Read the model definition and answer for the solid it produces. Units are mm, in the model's axes. Face numbers are marked on the shaded views. A direction names the side the tool comes from. Give positions to 0.01 mm unless a question says otherwise; leave off trailing zeros. Write each loop counter-clockwise with the first axis right and the second up, starting at its lowest first coordinate (ties: lowest second). Pieces come first, ordered by that corner, then holes. Notation, with made-up numbers: M -7.5,19 L 22.5,19 A31 ccw 22.5,43 Z; hole C -24.75,-7.5 d10. An arc over 180 degrees is marked long. Use a Markdown table: item, result. Add a question column.
Item 1: Consider probe 1 along Y at (x, z) = (0, 6) (3 decimals); probe 2 along Z at (x, y) = (0, -11.7) (3 decimals); probe 3 along Y at (x, z) = (-11.5, 8). Determine where each line is inside the solid, lowest interval first. Write a range as [from, to].
Item 2: Given P1, Ø2.5, axis at x = 0, z = 7.125, coming from the +Y side; P2, Ø3, axis at y = -7.5, z = 5.5, coming from the +X side; P3, Ø2.5, axis at x = -4.5, z = 6, coming from the -Y side; P4, Ø3, axis at x = -3.5, y = -8.5, coming from the -Z side, each flat-ended and moving along its own axis, determine where each tip first touches the part or whether it passes through.
Item 3: For the marked faces 4 and 5, determine the directions among +Z, -Z, +X, -X, +Y, -Y from which every point of the face is accessible in a straight line to the end or side of a thin tool.
Item 4: The mould has two halves that part along Z. Classify the marked faces 1, 2 and 3: pulls with the +Z half, pulls with the -Z half, needs draft (parallel to the pull), parting line crosses it, or undercut.
Item 5: A cutting plane is placed at A-A on x = 0. Determine the outline of the cut face in (y, z) (3 decimals).
Item 6: A cutting plane is placed at B-B on z = 5.5. Determine the outline of the cut face in (x, y) (3 decimals).
Item 7: A cutting plane is placed at D-D on y = -4. Determine the outline of the cut face in (x, z).
Item 8: A cutting plane is placed at C-C on y = -11.75. Determine the outline of the cut face in (x, z) (3 decimals).
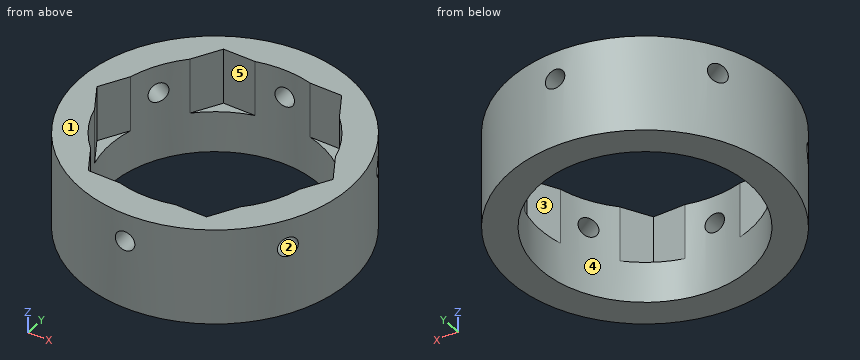
from build123d import *

# Parameters (mm, degrees)
SKETCH1_R               = 14
BOSS_EXTRUDE1_DEPTH     = 10
CUT_EXTRUDE1_REACH      = 24.181
SKETCH2_R               = 10.875
CUT_EXTRUDE2_DEPTH      = 5.75
CUT_EXTRUDE3_REACH      = 31.937
CUT_EXTRUDE3_END_RADIUS = 14
SKETCH4_R               = 1
CUT_EXTRUDE4_REACH      = 33.684
CUT_EXTRUDE4_END_RADIUS = 14
SKETCH5_R               = 1
CUT_EXTRUDE5_REACH      = 33.684
CUT_EXTRUDE5_END_RADIUS = 14
SKETCH6_R               = 1
CUT_EXTRUDE6_REACH      = 31.937
CUT_EXTRUDE6_END_RADIUS = 14
SKETCH7_R               = 1
CUT_EXTRUDE7_REACH      = 33.684
CUT_EXTRUDE7_END_RADIUS = 14
SKETCH8_R               = 1
CUT_EXTRUDE8_REACH      = 33.684
CUT_EXTRUDE8_END_RADIUS = 14
SKETCH9_R               = 1


with BuildPart() as part:
    # Sketch1 → Boss-Extrude1 (new body)
    with BuildSketch(Plane.XY):
        Circle(SKETCH1_R)
    extrude(amount=BOSS_EXTRUDE1_DEPTH)

    # Sketch2 → Cut-Extrude1 (cut, up to next)
    with BuildSketch(Plane.XY.offset(10), mode=Mode.PRIVATE) as cut_extrude1_sk1:
        Circle(SKETCH2_R)
    cut_extrude1_tool1 = extrude(cut_extrude1_sk1.sketch, amount=-CUT_EXTRUDE1_REACH, mode=Mode.PRIVATE) & part.part
    add(cut_extrude1_tool1.solids().sort_by_distance((0, 0, 10))[0], mode=Mode.SUBTRACT)

    # Sketch3 → Cut-Extrude2 (cut)
    with BuildSketch(Plane.XY.offset(10)):
        Polygon((12.124355653, 0), (6.062177826, 10.5), (-6.062177826, 10.5), (-12.124355653, 0), (-6.062177826, -10.5), (6.062177826, -10.5), align=None)
    extrude(amount=-CUT_EXTRUDE2_DEPTH, mode=Mode.SUBTRACT)

    # Cut-Extrude3: up to this cylinder (the profile starts inside it)
    cut_extrude3_end = Plane(origin=(0, 0, 7.125), z_dir=(0, 0, -1)) * Cylinder(CUT_EXTRUDE3_END_RADIUS, 92.874, mode=Mode.PRIVATE)
    # Sketch4 → Cut-Extrude3 (cut, up to the surface)
    with BuildSketch(Plane(origin=(0, 10.5, 0), x_dir=(-1, 0, 0), z_dir=(0, -1, 0)), mode=Mode.PRIVATE) as cut_extrude3_sk1:
        with Locations(Location((0, -7.125, 0), (0, 0, 180))):
            Circle(SKETCH4_R)
    cut_extrude3_tool1 = extrude(cut_extrude3_sk1.sketch, amount=-CUT_EXTRUDE3_REACH, mode=Mode.PRIVATE) & cut_extrude3_end
    add(cut_extrude3_tool1.solids().sort_by_distance((0, 10.5, 7.125))[0], mode=Mode.SUBTRACT)

    # Cut-Extrude4: up to this cylinder (the profile starts inside it)
    cut_extrude4_end = Plane(origin=(0, 0, 7.125), z_dir=(0, 0, -1)) * Cylinder(CUT_EXTRUDE4_END_RADIUS, 96.368, mode=Mode.PRIVATE)
    # Sketch5 → Cut-Extrude4 (cut, up to the surface)
    with BuildSketch(Plane(origin=(9.09326674, 5.25, 0), x_dir=(0, 0, 1), z_dir=(-0.8660254037844386, -0.4999999999999999, 0)), mode=Mode.PRIVATE) as cut_extrude4_sk1:
        with Locations(Location((7.125, 0, 0), (0, 0, 270))):
            Circle(SKETCH5_R)
    cut_extrude4_tool1 = extrude(cut_extrude4_sk1.sketch, amount=-CUT_EXTRUDE4_REACH, mode=Mode.PRIVATE) & cut_extrude4_end
    add(cut_extrude4_tool1.solids().sort_by_distance((9.093267, 5.25, 7.125))[0], mode=Mode.SUBTRACT)

    # Cut-Extrude5: up to this cylinder (the profile starts inside it)
    cut_extrude5_end = Plane(origin=(0, 0, 7.125), z_dir=(0, 0, -1)) * Cylinder(CUT_EXTRUDE5_END_RADIUS, 96.368, mode=Mode.PRIVATE)
    # Sketch6 → Cut-Extrude5 (cut, up to the surface)
    with BuildSketch(Plane(origin=(9.09326674, -5.25, 0), x_dir=(0, 0, 1), z_dir=(-0.8660254037844386, 0.5, 0)), mode=Mode.PRIVATE) as cut_extrude5_sk1:
        with Locations(Location((7.125, 0, 0), (0, 0, 270))):
            Circle(SKETCH6_R)
    cut_extrude5_tool1 = extrude(cut_extrude5_sk1.sketch, amount=-CUT_EXTRUDE5_REACH, mode=Mode.PRIVATE) & cut_extrude5_end
    add(cut_extrude5_tool1.solids().sort_by_distance((9.093267, -5.25, 7.125))[0], mode=Mode.SUBTRACT)

    # Cut-Extrude6: up to this cylinder (the profile starts inside it)
    cut_extrude6_end = Plane(origin=(0, 0, 7.125), z_dir=(0, 0, -1)) * Cylinder(CUT_EXTRUDE6_END_RADIUS, 92.874, mode=Mode.PRIVATE)
    # Sketch7 → Cut-Extrude6 (cut, up to the surface)
    with BuildSketch(Plane(origin=(0, -10.5, 0), x_dir=(1, 0, 0), z_dir=(0, 1, 0)), mode=Mode.PRIVATE) as cut_extrude6_sk1:
        with Locations((0, -7.125)):
            Circle(SKETCH7_R)
    cut_extrude6_tool1 = extrude(cut_extrude6_sk1.sketch, amount=-CUT_EXTRUDE6_REACH, mode=Mode.PRIVATE) & cut_extrude6_end
    add(cut_extrude6_tool1.solids().sort_by_distance((0, -10.5, 7.125))[0], mode=Mode.SUBTRACT)

    # Cut-Extrude7: up to this cylinder (the profile starts inside it)
    cut_extrude7_end = Plane(origin=(0, 0, 7.125), z_dir=(0, 0, -1)) * Cylinder(CUT_EXTRUDE7_END_RADIUS, 96.368, mode=Mode.PRIVATE)
    # Sketch8 → Cut-Extrude7 (cut, up to the surface)
    with BuildSketch(Plane(origin=(-9.09326674, -5.25, 0), x_dir=(0, 0, -1), z_dir=(0.8660254037844385, 0.5000000000000003, 0)), mode=Mode.PRIVATE) as cut_extrude7_sk1:
        with Locations(Location((-7.125, 0, 0), (0, 0, 270))):
            Circle(SKETCH8_R)
    cut_extrude7_tool1 = extrude(cut_extrude7_sk1.sketch, amount=-CUT_EXTRUDE7_REACH, mode=Mode.PRIVATE) & cut_extrude7_end
    add(cut_extrude7_tool1.solids().sort_by_distance((-9.093267, -5.25, 7.125))[0], mode=Mode.SUBTRACT)

    # Cut-Extrude8: up to this cylinder (the profile starts inside it)
    cut_extrude8_end = Plane(origin=(0, 0, 7.125), z_dir=(0, 0, -1)) * Cylinder(CUT_EXTRUDE8_END_RADIUS, 96.368, mode=Mode.PRIVATE)
    # Sketch9 → Cut-Extrude8 (cut, up to the surface)
    with BuildSketch(Plane(origin=(-9.09326674, 5.25, 0), x_dir=(0, 0, -1), z_dir=(0.8660254037844388, -0.49999999999999983, 0)), mode=Mode.PRIVATE) as cut_extrude8_sk1:
        with Locations(Location((-7.125, 0, 0), (0, 0, 270))):
            Circle(SKETCH9_R)
    cut_extrude8_tool1 = extrude(cut_extrude8_sk1.sketch, amount=-CUT_EXTRUDE8_REACH, mode=Mode.PRIVATE) & cut_extrude8_end
    add(cut_extrude8_tool1.solids().sort_by_distance((-9.093267, 5.25, 7.125))[0], mode=Mode.SUBTRACT)


solid = part.part
Filled in:
| question | item | result |
|---|---|---|
| 1 | probe 1 | [-14, -10.875], [10.875, 14] |
| 1 | probe 2 | [0, 6.125], [8.125, 10] |
| 1 | probe 3 | [-7.98, -7.2], [-6.08, -1.08], [1.08, 6.08], [7.2, 7.98] |
| 2 | P1 | y = 14 |
| 2 | P2 | x = 12.65 |
| 2 | P3 | y = -13.62 |
| 2 | P4 | through |
| 3 | face 4 | +Z, -Z |
| 3 | face 5 | +Z |
| 4 | face 1 | pulls with the +Z half |
| 4 | face 2 | undercut |
| 4 | face 3 | needs draft |
| 5 | outline | M -14,0 L -10.875,0 L -10.875,6.125 L -14,6.125 Z; M -14,8.125 L -10.875,8.125 L -10.875,10 L -14,10 Z; M 10.875,0 L 14,0 L 14,6.125 L 10.875,6.125 Z; M 10.875,8.125 L 14,8.125 L 14,10 L 10.875,10 Z |
| 6 | outline | C 0,0 d28; hole M -12.124,0 L -10.509,-2.798 A10.875 ccw -7.678,-7.702 L -6.062,-10.5 L -2.831,-10.5 A10.875 ccw 2.831,-10.5 L 6.062,-10.5 L 7.678,-7.702 A10.875 ccw 10.509,-2.798 L 12.124,0 L 10.509,2.798 A10.875 ccw 7.678,7.702 L 6.062,10.5 L 2.831,10.5 A10.875 ccw -2.831,10.5 L -6.062,10.5 L -7.678,7.702 A10.875 ccw -10.509,2.798 Z |
| 7 | outline | M -13.42,0 L -10.11,0 L -10.11,10 L -13.42,10 Z; M 10.11,0 L 13.42,0 L 13.42,10 L 10.11,10 Z |
| 8 | outline | M -7.612,0 L 7.612,0 L 7.612,10 L -7.612,10 Z; hole C 0,7.125 d2 |
